Read the model definition and answer for the solid it produces. Units are mm, in the model's axes. A direction names the side the tool comes from. Coordinates: 2 decimals unless noted, no trailing zeros. Write each loop counter-clockwise with the first axis right and the second up, starting at its lowest first coordinate (ties: lowest second). Pieces come first, ordered by that corner, then holes. Notation, with made-up numbers: (50, -38) -> (98, -38) arc R32 cw to (98, -10) -> close; hole circle Ø3 at (66, 57). An arc over 180 degrees is marked (long way). One line per item, written item: value. Start each with the question number.
1. Find section A-A, the plane z = -65. Write down the section's boundary in (x, y), and give its area (3 significant figures).
2. Given P1, Ø8, axis at y = 67, z = -113.5, coming from the -X side, flat-ended and moving along its own axis, determine where the tip first touches the part or whether it passes through.
3. For a pull along Z with two mould halves and no side action, classify faces 3 (the flat face through (0, 35, -2)), 4 (the flat face through (75, 64, -127)), 5 (the flat face through (149.86, 64, -63)) as pulls with the +Z half, pulls with the -Z half, needs draft (parallel to the pull), parting line crosses it, or undercut.
4. For faces 1 (the flat face through (75, 63, 0)), 2 (the flat face through (74, 64, -2.54)), determine the directions among +Z, -Z, +X, -X, +Y, -Y from which every point of the face is accessible in a straight line to the end or side of a thin tool.
5. Find section D-D, the plane z = -34.5. Write down the section's boundary in (x, y), and give its area (3 significant figures).
6. Consider line 1 along Z through (x, y) = (129.5, 78.5); line 2 along Y through (x, z) = (111, -28); line 3 along X through (y, z) = (119, -8.5). Determine where each line is inside the solid, lowest interval first.
7. Find section B-B, the plane x = 104.5. Write down the section's boundary in (y, z).
8. Find section C-C, the plane y = 39. Write down the section's boundary in (x, z).
Autodesk Inventor part; units mm, degrees
ref_plane "YZ Plane" through (0, 0, 0) normal (1, 0, 0) x (0, 1, 0)
ref_plane "XZ Plane" through (0, 0, 0) normal (0, 1, 0) x (-1, 0, 0)
ref_plane "XY Plane" through (0, 0, 0) normal (0, 0, 1) x (1, 0, 0)
sketch "Sketch1" plane through (0, 0, 0) normal (1, 0, 0) x (0, 1, 0)
  line L0 (0, 0) -> (127, 0)
  line L1 (127, 0) -> (127, -127)
  line L2 (127, -127) -> (0, -127)
  line L3 (0, -127) -> (0, 0)
  line L4 (127, -127) -> (124.46, -127)
  line L5 (124.46, -127) -> (124.46, -124.46)
  line L6 (124.46, -124.46) -> (127, -124.46)
  line L7 (127, -124.46) -> (127, -127)
  line L8 (127, 0) -> (124.46, 0)
  line L9 (124.46, 0) -> (124.46, -2.54)
  line L10 (124.46, -2.54) -> (127, -2.54)
  line L11 (127, -2.54) -> (127, 0)
  line L12 (124.46, -2.54) -> (2.54, -2.54)
  line L13 (2.54, -2.54) -> (2.54, -124.46)
  line L14 (2.54, -124.46) -> (124.46, -124.46)
  line L15 (124.46, -124.46) -> (124.46, -2.54)
  line L16 (124.46, -124.46) -> (122.682, -124.46)
  line L17 (124.46, -2.54) -> (68.58, -2.54)
  line L18 (124.46, -4.572) -> (124.46, -2.54)
  line L19 (0, 0) -> (50.8, 0)
  line L20 (0, -25.4) -> (0, 0)
  line L21 (127, 0) -> (76.2, 0)
  line L22 (127, -25.4) -> (127, 0)
extrude "Extrusion1" add sketch "Sketch1" along normal blind 152.4
extrude "Extrusion2" cut sketch "Sketch1" along normal blind 149.86 contours L15 L14 L13 L12
sketch "Sketch10" plane through (0, 2.54, -124.46) normal (0, 0, 1) x (1, 0, 0)
  line L0 (0, 0) -> (149.86, 0)
  line L1 (149.86, 0) -> (90.17, 0)
  line L2 (90.17, 0) -> (90.17, 2.032)
  line L3 (90.17, 2.032) -> (149.86, 2.032)
  line L4 (149.86, 2.032) -> (149.86, 0)
  line L5 (0, 0) -> (90.17, 2.032)
  point P0 (0, -2.54)
  dimension "d22" = 59.69
  dimension "d23" = 2.032
extrude "Extrusion5" add sketch "Sketch10" along normal blind 121.92
sketch "Sketch11" plane through (0, 127, 0) normal (0, 1, 0) x (1, 0, 0)
  line L0 (0, 0) -> (152.4, 0)
  line L1 (152.4, 0) -> (121.92, 0)
  line L2 (121.92, 0) -> (121.92, 50.8)
  line L3 (121.92, 50.8) -> (152.4, 50.8)
  line L4 (152.4, 50.8) -> (152.4, 0)
  line L5 (152.4, 126.0289) -> (121.92, 126.0289)
  line L6 (121.92, 126.0289) -> (121.92, 75.2289)
  line L7 (121.92, 75.2289) -> (152.4, 75.2289)
  line L8 (152.4, 75.2289) -> (152.4, 126.0289)
  line L9 (121.92, 75.2289) -> (106.68, 75.2289)
  line L10 (106.68, 75.2289) -> (106.68, 50.8)
  line L11 (106.68, 50.8) -> (121.92, 50.8)
  line L12 (121.92, 50.8) -> (121.92, 75.2289)
  dimension "d30" = 30.48
  dimension "d31" = 50.8
  dimension "d32" = 30.48
  dimension "d33" = 50.8
  dimension "d34" = 15.24
extrude "Extrusion6" cut sketch "Sketch11" against normal blind 2.54 contours L11 L10 L9 L12
properties part number "box-1"
Answer block:
1. outline: (0, 0) -> (152.4, 0) -> (152.4, 127) -> (121.92, 127) -> (121.92, 124.46) -> (149.86, 124.46) -> (149.86, 4.57) -> (90.17, 4.57) -> (0, 2.54) -> close; (0, 124.46) -> (106.68, 124.46) -> (106.68, 127) -> (0, 127) -> close
1. area: 1,260 mm2
2. P1: stops at x = 149.86
3. face 3: needs draft
3. face 4: pulls with the -Z half
3. face 5: undercut
4. face 1: +Z, +X, -X, +Y, -Y
4. face 2: -X
5. outline: (0, 0) -> (152.4, 0) -> (152.4, 127) -> (0, 127) -> (0, 124.46) -> (149.86, 124.46) -> (149.86, 4.57) -> (90.17, 4.57) -> (0, 2.54) -> close
5. area: 1,300 mm2
6. line 1: z = -127 to -124.46, -2.54 to 0
6. line 2: y = 0 to 4.57, 124.46 to 127
6. line 3: x = 149.86 to 152.4
7. outline: (0, -127) -> (127, -127) -> (127, 0) -> (0, 0) -> close; hole (4.57, -124.46) -> (124.46, -124.46) -> (124.46, -2.54) -> (4.57, -2.54) -> close
8. outline: (0, -127) -> (152.4, -127) -> (152.4, 0) -> (0, 0) -> (0, -2.54) -> (149.86, -2.54) -> (149.86, -124.46) -> (0, -124.46) -> close
